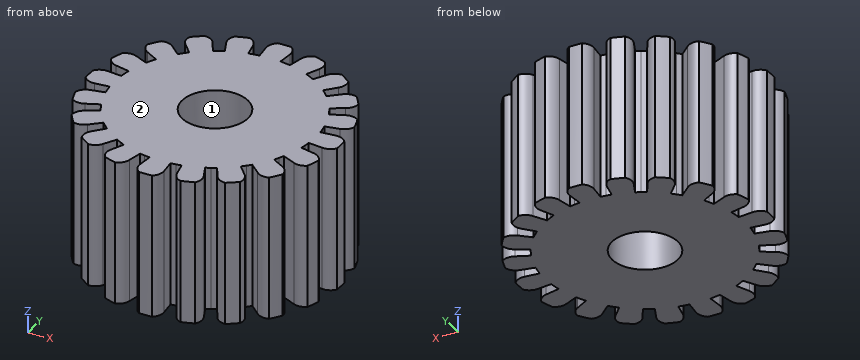
from build123d import *

# Parameters (mm, degrees)
BOSS_EXTRUDE3_DEPTH     = 22
CIRPATTERN3_COUNT       = 20
SKETCH2_R               = 10
CUT_EXTRUDE1_DEPTH      = 23
CUT_EXTRUDE1_DEPTH_BACK = 23


with BuildPart() as part:
    # Sketch1 → Boss-Extrude3 (new body, symmetric)
    with BuildSketch(Plane.XY):
        with BuildLine():
            Line((34.808266338, 3.658496214), (30.432369998, 3.198570976))
            ThreePointArc((30.432369998, 3.198570976), (30.338212758, 3.994101482), (30.223263222, 4.78689463))
            Line((30.223263222, 4.78689463), (0, 0))
            Line((0, 0), (30.223263222, -4.78689463))
            ThreePointArc((30.223263222, -4.78689463), (30.338212758, -3.994101482), (30.432369998, -3.198570976))
            Line((30.432369998, -3.198570976), (34.808266338, -3.658496214))
            ThreePointArc((34.808266338, -3.658496214), (36.855171385, -3.340239675), (38.447237088, -2.014934315))
            ThreePointArc((38.447237088, -2.014934315), (38.5, 0), (38.447237088, 2.014934315))
            ThreePointArc((38.447237088, 2.014934315), (36.855171385, 3.340239675), (34.808266338, 3.658496214))
        make_face()
    boss_extrude3 = extrude(amount=BOSS_EXTRUDE3_DEPTH, both=True)

    # CirPattern3: Boss-Extrude3 ×20 about axis
    cirpattern3_axis = Axis((0, 0, 0), (0, 0, 1))
    for i in range(1, CIRPATTERN3_COUNT):
        add(boss_extrude3.rotate(cirpattern3_axis, i * 360 / CIRPATTERN3_COUNT))

    # Sketch2 → Cut-Extrude1 (cut, two sides)
    with BuildSketch(Plane.XY) as cut_extrude1_sk:
        Circle(SKETCH2_R)
    extrude(amount=CUT_EXTRUDE1_DEPTH, mode=Mode.SUBTRACT)
    extrude(cut_extrude1_sk.sketch, amount=-CUT_EXTRUDE1_DEPTH_BACK, mode=Mode.SUBTRACT)


solid = part.part
CAD build for the part. Positions are in the model's coordinates, mm. Face numbers are marked on the shaded views. Round coordinates to 2 decimals unless told otherwise and drop trailing zeros. Loops run counter-clockwise (first coordinate to the right, second up) from the corner with the lowest first, then second, coordinate; pieces in that order, holes last.
(1) Cut at A-A (y = 0). Give the cut face in (x, z).
(2) Wall check: line 1 along X through (y, z) = (14, -6); line 2 along X through (y, z) = (-28, 0.5); line 3 along Y through (x, z) = (29, -9). Give the ranges that are in metal, low to high.
(3) Drop flat-ended pins along their axis: pin 1 (3 mm diameter, centred on x = 23.5, z = 2.5, fed in from -Y); pin 2 (3 mm diameter, centred on x = -11, z = -8.5, fed in from -Y); pin 3 (5 mm diameter, centred on y = -8, z = -9.5, fed in from -X). Give the stop position or say it passes through.
(4) Two-plate mould, pull along Y, no slides. Class the marked faces 1 and 2: +Y half, -Y half, draft (parallel to the pull), parting line (faces both ways), or undercut.
Findings below:
1. outline: (-38.5, -22) - (-10, -22) - (-10, 22) - (-38.5, 22) - close; (10, -22) - (38.5, -22) - (38.5, 22) - (10, 22) - close
2. line 1: x = -35.65 to -31.44, -27.21 to 27.21, 31.44 to 35.65
2. line 2: x = -24.39 to -16.17, -12.47 to 12.47, 16.17 to 24.39
2. line 3: y = -24.43 to -16.74, -12.91 to 12.91, 16.74 to 24.43
3. pin 1: stops at y = -31.6
3. pin 2: stops at y = -37.19
3. pin 3: stops at x = -37.19
4. face 1: undercut
4. face 2: draft
